Can you work these out from the model? Positions are in its coordinate system, mm. Give positions to 0.01 mm unless a question says otherwise; leave off trailing zeros. Write each loop counter-clockwise with the first axis right and the second up, starting at its lowest first coordinate (ties: lowest second). Pieces come first, ordered by that corner, then holes.
1. Suppose I cut it at B-B (x = -50.8). Please give me the cut outline in (y, z) (3 decimals), and give its area (3 significant figures).
2. I'm going to push flat-ended pins straight in: pin 1 (1.5 mm diameter, centred on x = 41, y = 2, fed in from +Z); pin 2 (3 mm diameter, centred on x = 11.314, z = 0, fed in from -Y). Where does each tip first touch, or does it pass through?
3. Suppose I cut it at D-D (z = -45). Please give me the cut outline in (x, y) (3 decimals), and give its area (3 significant figures).
4. Thinking about a two-plate mould opening in Z: for faces 1 (the cylindrical face through (-46.367, 1.565, -60.47)), 2 (the cylindrical face through (9.36, 1.61, -0.43)), 3 (the flat face through (1, 3.175, 16)), which applies, pulls with the +Z half, pulls with the -Z half, needs draft (parallel to the pull), parting line crosses it, or undercut?
5. If I drill on probe 1 along X at (y, z) = (1.85, 0) (3 decimals); probe 2 along X at (y, z) = (1.7, 5.5); probe 3 along Z at (x, y) = (-49, 2.4), over which ranges is the centre line in solid material (lowest first)?
6. Suppose I cut it at A-A (z = 0). Please give me the cut outline in (x, y) (3 decimals).
7. Suppose I cut it at C-C (y = 1.9). Give the number of separate pieces and of enclosed holes in the cut face, and give its area (3 significant figures).
```python
from build123d import *

# Parameters (mm, degrees)
SKETCH1_R           = 76.2
BOSS_EXTRUDE1_DEPTH = 3.175
SKETCH2_R           = 7
CUT_EXTRUDE1_DEPTH  = 108.809835474
SKETCH3_R           = 2
CUT_EXTRUDE2_DEPTH  = 108.809835474
SKETCH4_R           = 3.175
CUT_EXTRUDE3_DEPTH  = 108.809835474
CUT_EXTRUDE4_REACH  = 109.81
SKETCH5_R           = 6.35


with BuildPart() as part:
    # Sketch1 → Boss-Extrude1 (new body)
    with BuildSketch(Plane(origin=(0, 0, 0), x_dir=(1, 0, 0), z_dir=(0, 1, 0))):
        with Locations(Location((0, 0, 0), (0, 0, 270))):
            Circle(SKETCH1_R)
    extrude(amount=BOSS_EXTRUDE1_DEPTH)

    # Sketch2 → Cut-Extrude1 (cut, through all)
    with BuildSketch(Plane(origin=(0, 3.175, 0), x_dir=(1, 0, 0), z_dir=(0, 1, 0))):
        with Locations(Location((0, 0, 0), (0, 0, 270))):
            Circle(SKETCH2_R)
    extrude(amount=-CUT_EXTRUDE1_DEPTH, mode=Mode.SUBTRACT)

    # Sketch3 → Cut-Extrude2 (cut, through all)
    with BuildSketch(Plane(origin=(0, 3.175, 0), x_dir=(1, 0, 0), z_dir=(0, 1, 0))):
        with Locations(Location((11.314, 0, 0), (0, 0, 270))):
            Circle(SKETCH3_R)
        with Locations(Location((0, -11.314, 0), (0, 0, 270))):
            Circle(SKETCH3_R)
        with Locations(Location((-11.314, 0, 0), (0, 0, 270))):
            Circle(SKETCH3_R)
        with Locations(Location((0, 11.314, 0), (0, 0, 270))):
            Circle(SKETCH3_R)
    extrude(amount=-CUT_EXTRUDE2_DEPTH, mode=Mode.SUBTRACT)

    # Sketch4 → Cut-Extrude3 (cut, through all)
    with BuildSketch(Plane.XZ):
        with Locations(Location((-50.8, 0, 0), (0, 0, 270))):
            Circle(SKETCH4_R)
        with Locations(Location((50.8, 0, 0), (0, 0, 270))):
            Circle(SKETCH4_R)
    extrude(amount=-CUT_EXTRUDE3_DEPTH, mode=Mode.SUBTRACT)

    # Sketch5 → Cut-Extrude4 (cut, up to next)
    with BuildSketch(Plane(origin=(0, 3.175, 0), x_dir=(1, 0, 0), z_dir=(0, 1, 0)), mode=Mode.PRIVATE) as cut_extrude4_sk1:
        with Locations(Location((0, 41.73382544, 0), (0, 0, 270))):
            Circle(SKETCH5_R)
    cut_extrude4_tool1 = extrude(cut_extrude4_sk1.sketch, amount=-CUT_EXTRUDE4_REACH, mode=Mode.PRIVATE) & part.part
    add(cut_extrude4_tool1.solids().sort_by_distance((0, 3.175, -41.733825))[0], mode=Mode.SUBTRACT)


solid = part.part
```
Checks:
1. outline: (0, -56.796) - (3.175, -56.796) - (3.175, -3.175) - (0, -3.175) - close; (0, 3.175) - (3.175, 3.175) - (3.175, 56.796) - (0, 56.796) - close
1. area: 340 mm2
2. pin 1: stops at z = 64.7
2. pin 2: passes through
3. outline: (-61.493, 0) - (-5.446, 0) - (-5.446, 3.175) - (-61.493, 3.175) - close; (5.446, 0) - (61.493, 0) - (61.493, 3.175) - (5.446, 3.175) - close
3. area: 356 mm2
4. face 1: parting line crosses it
4. face 2: undercut
4. face 3: needs draft
5. probe 1: x = -76.2 to -53.975, -47.625 to -13.314, -9.314 to -7, 7 to 9.314, 13.314 to 47.625, 53.975 to 76.2
5. probe 2: x = -76 to -4.33, 4.33 to 76
5. probe 3: z = -58.36 to -2.62, 2.62 to 58.36
6. outline: (-76.2, 0) - (-53.975, 0) - (-53.975, 3.175) - (-76.2, 3.175) - close; (-47.625, 0) - (-13.314, 0) - (-13.314, 3.175) - (-47.625, 3.175) - close; (-9.314, 0) - (-7, 0) - (-7, 3.175) - (-9.314, 3.175) - close; (7, 0) - (9.314, 0) - (9.314, 3.175) - (7, 3.175) - close; (13.314, 0) - (47.625, 0) - (47.625, 3.175) - (13.314, 3.175) - close; (53.975, 0) - (76.2, 0) - (76.2, 3.175) - (53.975, 3.175) - close
7. separate pieces: 1
7. enclosed holes: 8
7. area: 17,800 mm2
